from build123d import *

# Parameters (mm, degrees)
F1_DEPTH  = 9
F2_W      = 130.0831899747
F2_H      = 3
F3_DEPTH  = 13
F4_DEPTH  = 25
F5_W      = 24
F5_H      = 2
F6_DEPTH  = 3
F8_R      = 3
F9_DEPTH  = 4
F7_W      = 24
F7_H      = 1
F7_W_2    = 93.5030970573
F10_DEPTH = 10
F11_DEPTH = 25
F12_R     = 5
F13_R     = 7


with BuildPart() as f1:
    # F0 (on Top) → F1 (new body)
    with BuildSketch(Plane.XY):
        Polygon((-64.5, 4.5), (-67.5, 4.5), (-67.5, -11.5), (67.5, -11.5), (67.5, 4.5), (-34.5, 4.5), align=None)
        Polygon((-34.5, 4.5), (-50.5, 11.5), (-64.5, 4.5), align=None)
    extrude(amount=F1_DEPTH)

    # F2 (on face) → F3 (cut)
    with BuildSketch(Plane(origin=(0, 4.5, 0), x_dir=(-1, 0, 0), z_dir=(0, 1, 0))):
        with Locations((0.6519891322, 4.4357408187)):
            Rectangle(F2_W, F2_H)
    extrude(amount=-F3_DEPTH, mode=Mode.SUBTRACT)

    # F4 (cut): a face of the model
    f4_faces = [f1.faces().sort_by_distance(p)[0] for p in [
        (-0.6519891322, -8.5, 4.4357408187),
    ]]
    extrude(f4_faces, amount=F4_DEPTH, mode=Mode.SUBTRACT)

    # F5 (on face) → F6 (join)
    with BuildSketch(Plane(origin=(0, 0, 5.9357408187), x_dir=(1, 0, 0), z_dir=(0, 0, -1))):
        with Locations((40.5, -3.5)):
            Rectangle(F5_W, F5_H)
    extrude(amount=F6_DEPTH)

    # F8 (on face) → F9 (join)
    with BuildSketch(Plane(origin=(0, 0, 5.9357408187), x_dir=(1, 0, 0), z_dir=(0, 0, -1))):
        with Locations((-50.5, -5.5)):
            Circle(F8_R)
    extrude(amount=F9_DEPTH)

    # F7 (on face) → F10 (cut)
    with BuildSketch(Plane(origin=(0, 4.5, 0), x_dir=(-1, 0, 0), z_dir=(0, 1, 0))):
        with Locations((-40.5, 4.4357408187)):
            Rectangle(F7_W, F7_H)
        with Locations((18.2515485287, 4.4357408187)):
            Rectangle(F7_W_2, F7_H)
    extrude(amount=-F10_DEPTH, mode=Mode.SUBTRACT)

    # F7 (on face) → F11 (cut)
    with BuildSketch(Plane(origin=(0, 4.5, 0), x_dir=(-1, 0, 0), z_dir=(0, 1, 0))):
        with Locations((18.2515485287, 4.4357408187)):
            Rectangle(F7_W_2, F7_H)
    extrude(amount=F11_DEPTH, mode=Mode.SUBTRACT)

    # F12
    f12_edges = [f1.edges().sort_by_distance(p)[0] for p in [
        (-50.5, 11.5, 1.46787),
        (-50.5, 11.5, 7.46787),
    ]]
    fillet(f12_edges, radius=F12_R)

    # F13
    f13_edges = [f1.edges().sort_by_distance(p)[0] for p in [
        (-67.5, -11.5, 4.5),
        (67.5, -11.5, 4.5),
    ]]
    fillet(f13_edges, radius=F13_R)


solid = f1.part
The listing builds one solid part. Answer for the finished solid, in the listing's coordinates (mm). A direction names the side the tool comes from. Round coordinates to 2 decimals unless told otherwise and drop trailing zeros. Order: outer loops, then holes, each group sorted by start corner. A loop starts at its lowest first (then second) coordinate and runs counter-clockwise, first axis right, second up. Notation, with made-up numbers: (14, 25) - (48, 25) arc R35 cw to (48, 60) - close; hole circle Ø1 at (24, 29.25). An arc over 180 degrees is marked (long way). Write item = value, one per line. Start each with the question number.
1) For faces 5 (the flat face through (-65.694, -2, 4)), 6 (the flat face through (17.2, 4.5, 6.4)), 7 (the cylindrical face through (-53.5, 5.4, 5.4)), determine the directions among +Z, -Z, +X, -X, +Y, -Y from which every point of the face is accessible in a straight line to the end or side of a thin tool.
2) For a pull along Y with two mould halves and no side action, classify faces 1 (the flat face through (0, -1, 5.936)), 2 (the flat face through (64.39, -2, 4)), 3 (the flat face through (0, -1, 2.936)), 4 (the cylindrical face through (65.5, -9.4, 4.6)) as released by +Y, released by -Y, zero draft, split by the parting line, or undercut.
3) Given pin 1 (2.5 mm diameter, centred on x = 1.5, z = 5.5, fed in from +Y), flat-ended and moving along its own axis, determine where the tip first touches the part or whether it passes through.
4) Straight lines are drawn through the part: L1, parallel to Z at x = 19, y = 0.75; L2, parallel to Z at x = -52, y = 6.25; L3, parallel to Y at x = -1.5, z = 2.5. For each, find the intervals that lie inside material, in ascending order.
5) Section B-B, the plane x = 23.5 is taken. Write down the section's boundary in (y, z), plus the area to 3 significant figures.
6) Section C-C, the plane x = -50.5 is taken. Write down the section's boundary in (y, z), plus the area to 3 significant figures.
7) Section A-A, the plane y = -2 is taken. Write down the section's boundary in (x, z).
Results list:
q1.face_5 = +Y
q1.face_6 = +Z, -Z, +X, +Y
q1.face_7 = none
q2.face_1 = undercut
q2.face_2 = zero draft
q2.face_3 = undercut
q2.face_4 = released by -Y
q3.pin_1 = 4.5
q4.L1 = 0 to 2.94, 5.94 to 9
q4.L2 = 0 to 3.94, 4.94 to 9
q4.L3 = -11.5 to 4.5
q5.outline = (-11.5, 0) - (4.5, 0) - (4.5, 2.94) - (-8.5, 2.94) - (-8.5, 5.94) - (4.5, 5.94) - (4.5, 9) - (-11.5, 9) - close
q5.area = 105 mm^2
q6.outline = (-11.5, 0) - (10.98, 0) - (10.98, 2.94) - (8.5, 2.94) - (8.5, 3.94) - (2.5, 3.94) - (2.5, 2.94) - (-8.5, 2.94) - (-8.5, 5.94) - (2.5, 5.94) - (2.5, 4.94) - (8.5, 4.94) - (8.5, 5.94) - (10.98, 5.94) - (10.98, 9) - (-11.5, 9) - close
q6.area = 156 mm^2
q7.outline = (-67.5, 0) - (67.5, 0) - (67.5, 9) - (-67.5, 9) - close; hole (-65.69, 2.94) - (64.39, 2.94) - (64.39, 5.94) - (-65.69, 5.94) - close
